from build123d import *

# Parameters (mm, degrees)
BOSS_EXTRUDE2_DEPTH     = 9.7
CUT_EXTRUDE1_DEPTH      = 26.804010416
CUT_EXTRUDE1_DEPTH_BACK = 26.804010416
SKETCH4_W               = 15.4
SKETCH4_H               = 15.4
CUT_EXTRUDE2_DEPTH      = 26.804010416
CUT_EXTRUDE2_DEPTH_BACK = 26.804010416
SKETCH5_R               = 2.7


with BuildPart() as part:
    # Sketch3 → Boss-Extrude2 (new body)
    with BuildSketch(Plane(origin=(0, 0, 0), x_dir=(1, 0, 0), z_dir=(0, 1, 0))):
        with BuildLine():
            Line((-17.904307086, 15.849061213), (17.904307086, 15.849061213))
            Line((17.904307086, 15.849061213), (17.549718608, 1.948996904))
            ThreePointArc((17.549718608, 1.948996904), (16.946433835, 0.56786764), (15.550369043, 0))
            Line((15.550369043, 0), (-15.550369043, 0))
            ThreePointArc((-15.550369043, 0), (-16.946433835, 0.56786764), (-17.549718608, 1.948996904))
            Line((-17.549718608, 1.948996904), (-17.904307086, 15.849061213))
        make_face()
    extrude(amount=BOSS_EXTRUDE2_DEPTH)

    # Sketch4 → Cut-Extrude1 (cut, two sides: drawn at the far end of the back side and taken through both)
    with BuildSketch(Plane.XY.offset(-CUT_EXTRUDE1_DEPTH_BACK)):
        with Locations((0, 10.7)):
            Rectangle(SKETCH4_W, SKETCH4_H)
    extrude(amount=CUT_EXTRUDE1_DEPTH + CUT_EXTRUDE1_DEPTH_BACK, mode=Mode.SUBTRACT)

    # Sketch5 → Cut-Extrude2 (cut, two sides: drawn at the far end of the back side and taken through both)
    with BuildSketch(Plane(origin=(0, 9.7, 0), x_dir=(1, 0, 0), z_dir=(0, 1, 0)).offset(-CUT_EXTRUDE2_DEPTH_BACK)):
        with Locations(Location((-12.701076771, 7.924530607, 0), (0, 0, 270))):
            Circle(SKETCH5_R)
        with Locations(Location((12.701076771, 7.924530607, 0), (0, 0, 270))):
            Circle(SKETCH5_R)
    extrude(amount=CUT_EXTRUDE2_DEPTH + CUT_EXTRUDE2_DEPTH_BACK, mode=Mode.SUBTRACT)


solid = part.part
Geometry check sheet. Reference: the model listing, model coordinates, mm. A direction names the side the tool comes from. Give positions to 0.01 mm unless a question says otherwise; leave off trailing zeros. Loops run counter-clockwise (first coordinate to the right, second up) from the corner with the lowest first, then second, coordinate; pieces in that order, holes last. Notation, with made-up numbers: M 49,0.25 L 78,0.25 A25 cw 78,28.25 Z; hole C 71.5,72 d1. An arc over 180 degrees is marked long. Answer as a JSON object with one key per item and string values. Group by question number.
Item 1: Access from +Z, -Z, +X, -X, +Y, -Y to the whole of each face (thin tool, end or side, straight path). Record for faces 1 (the flat face through (-0.3, 2.6, -15.849)), 2 (the flat face through (-7.7, 6, -8)).
Item 2: Sectioned sample at B-B on x = 12. Record the boundary of the cut face in (y, z), plus the area to 3 significant figures.
Item 3: Sectioned sample at D-D on y = 2. Record the boundary of the cut face in (x, z), plus the area to 3 significant figures.
Item 4: Material ranges on L1, parallel to X at y = 3.5, z = -5.75; L2, parallel to X at y = 9.25, z = -6.5; L3, parallel to X at y = 1.75, z = -7, recorded low to high.
Item 5: Sectioned sample at C-C on z = -7.75. Record the boundary of the cut face in (x, y), plus the area to 3 significant figures.
Item 6: Mould release check, pull along Z, two halves, no side actions. Record for faces 3 (the cylindrical face through (-13.735, 4.782, -5.43)), 4 (the cylindrical face through (16.96, 4.78, -0.58)), 5 (the flat face through (7.7, 6, -8)): pulls with the +Z half, pulls with the -Z half, needs draft (parallel to the pull), parting line crosses it, or undercut.
Item 7: Gauge pin test, flat ends, axial feed: pin 1 (1 mm diameter, centred on y = 5, z = -8.5, fed in from +X); pin 2 (4 mm diameter, centred on x = 5, z = -4.5, fed in from +Y); pin 3 (4 mm diameter, centred on y = 1, z = -1.5, fed in from +X). Record the tip position at first contact, or that the pin passes through.
Item 8: Sectioned sample at A-A on y = 3.75. Record the boundary of the cut face in (x, z), plus the area to 3 significant figures.
Findings below:
{
 "1": {"face 1": "-Z, +X, -X, +Y, -Y", "face 2": "+Z, -Z, +Y"},
 "2": {"outline": "M 0,-15.85 L 9.7,-15.85 L 9.7,-10.53 L 0,-10.53 Z; M 0,-5.32 L 9.7,-5.32 L 9.7,0 L 0,0 Z", "area": "103 mm2"},
 "3": {"outline": "M -17.9,-15.85 L 17.9,-15.85 L 17.55,-1.95 A2 ccw 15.55,0 L -15.55,0 A2 ccw -17.55,-1.95 Z; hole C -12.7,-7.92 d5.4; hole C 12.7,-7.92 d5.4", "area": "514 mm2"},
 "4": {"L1": "-17.65 to -14.3, -11.1 to -7.7, 7.7 to 11.1, 14.3 to 17.65", "L2": "-17.67 to -14.99, -10.41 to -7.7, 7.7 to 10.41, 14.99 to 17.67", "L3": "-17.68 to -15.24, -10.16 to 10.16, 15.24 to 17.68"},
 "5": {"outline": "M -17.7,0 L -15.4,0 L -15.4,9.7 L -17.7,9.7 Z; M -10.01,0 L 10.01,0 L 10.01,9.7 L 7.7,9.7 L 7.7,3 L -7.7,3 L -7.7,9.7 L -10.01,9.7 Z; M 15.4,0 L 17.7,0 L 17.7,9.7 L 15.4,9.7 Z", "area": "136 mm2"},
 "6": {"face 3": "undercut", "face 4": "pulls with the +Z half", "face 5": "needs draft"},
 "7": {"pin 1": "x = 17.73", "pin 2": "y = 3", "pin 3": "x = 17.59"},
 "8": {"outline": "M -17.9,-15.85 L -7.7,-15.85 L -7.7,0 L -15.55,0 A2 ccw -17.55,-1.95 Z; M 7.7,-15.85 L 17.9,-15.85 L 17.55,-1.95 A2 ccw 15.55,0 L 7.7,0 Z; hole C -12.7,-7.92 d5.4; hole C 12.7,-7.92 d5.4", "area": "270 mm2"}
}
